Design review of the part built by this model. Coordinates are the model's own, in mm. Round coordinates to 2 decimals unless told otherwise and drop trailing zeros. Loops run counter-clockwise (first coordinate to the right, second up) from the corner with the lowest first, then second, coordinate; pieces in that order, holes last. Notation, with made-up numbers: (28, 83) - (87, 83) arc R10 cw to (87, 93) - close; hole circle Ø5 at (31.5, -34). An arc over 180 degrees is marked (long way). Answer as CSV lines item,"result". Start each with the question number.
(1) Consider section B-B (z = 2). Give the boundary of the cut face in (x, y), and give its area (3 significant figures).
(2) Wall thickness on L1, parallel to Y at x = 14, z = 9.25; L2, parallel to Y at x = 66, z = 6.25: over which ranges is each line inside the solid? List them lowest first.
(3) For P1, Ø6, axis at x = 86.5, z = 1.5, coming from the +Y side, flat-tipped, find the tip position at first contact; note if it passes through.
from build123d import *

# Parameters (mm, degrees)
ESQUISSE1_W        = 125
ESQUISSE1_H        = 130
BOSS_EXTRU_1_DEPTH = 10
CHANFREIN1_SIZE2   = 7.002075382
CHANFREIN1_SIZE    = 10


with BuildPart() as part:
    # Esquisse1 → Boss.-Extru.1 (new body)
    with BuildSketch(Plane.XY):
        with Locations((62.5, 65)):
            Rectangle(ESQUISSE1_W, ESQUISSE1_H)
    extrude(amount=BOSS_EXTRU_1_DEPTH)

    # Chanfrein1
    chanfrein1_edges = [part.edges().sort_by_distance(p)[0] for p in [
        (62.5, 130, 0),
    ]]
    chanfrein1_side = [part.faces().sort_by_distance(p)[0] for p in [
        (62.5, 130, 0.140041508),
    ]]
    chamfer(chanfrein1_edges, length=CHANFREIN1_SIZE - 0.0001, length2=CHANFREIN1_SIZE2 - 0.0001, reference=chanfrein1_side[0])  # a hair under: the kernel refuses the full size


solid = part.part
Determined:
1,outline,"(0, 0) - (125, 0) - (125, 124.4) - (0, 124.4) - close"
1,area,"15,500 mm^2"
2,L1,"y = 0 to 129.47"
2,L2,"y = 0 to 127.37"
3,P1,"stops at y = 126.15"
